Source: CAD feature listing. Evaluate the final solid. Frame: model axes, mm. Face numbers are marked on the shaded views. A direction names the side the tool comes from. Coordinates: 2 decimals unless noted, no trailing zeros. Order: outer loops, then holes, each group sorted by start corner. A loop starts at its lowest first (then second) coordinate and runs counter-clockwise, first axis right, second up.
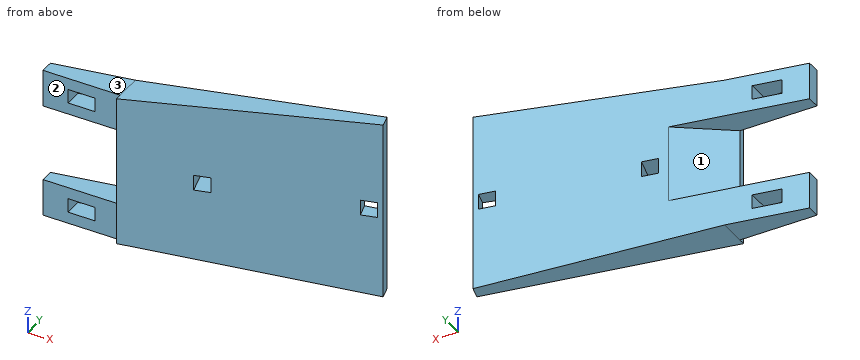
```python
from build123d import *

# Parameters (mm, degrees)
SALIENTE_EXTRUIR1_DEPTH     = 70
CORTAR_EXTRUIR1_START       = -26.44505645
CORTAR_EXTRUIR1_OUTLINE_W   = 30
CORTAR_EXTRUIR1_OUTLINE_H   = 30
CORTAR_EXTRUIR1_OUTLINE_W_2 = 10.5
CORTAR_EXTRUIR1_OUTLINE_H_2 = 5.5
CORTAR_EXTRUIR1_DEPTH       = 28.94505645
CROQUIS3_W                  = 6
CROQUIS3_H                  = 6
CORTAR_EXTRUIR2_DEPTH       = 118.634247959
CORTAR_EXTRUIR3_DEPTH       = 15
CORTAR_EXTRUIR3_DEPTH_BACK  = 15


# Read off the part's stored shape, not the designer's step: Cortar-Extruir1
with BuildPart() as part:
    # Croquis1 → Saliente-Extruir1 (new body)
    with BuildSketch(Plane.XY):
        Polygon((0, 0), (90, 24.115427319), (88.705904774, 28.94505645), (-30, 7.5), (-30, 2.5), (0, 2.5), align=None)
    extrude(amount=SALIENTE_EXTRUIR1_DEPTH)

    # Cortar-Extruir1 outline → Cortar-Extruir1 (cut)
    with BuildSketch(Plane.XZ.offset(-2.5).offset(CORTAR_EXTRUIR1_START)):
        Polygon((90, 0), (0, 5.5), (-30, 5.5), (-30, 0), align=None)
        with Locations((-15, 35)):
            Rectangle(CORTAR_EXTRUIR1_OUTLINE_W, CORTAR_EXTRUIR1_OUTLINE_H)
        Polygon((-30, 64.5), (0, 64.5), (90, 70), (-30, 70), align=None)
        with Locations((-15, 12.75)):
            Rectangle(CORTAR_EXTRUIR1_OUTLINE_W_2, CORTAR_EXTRUIR1_OUTLINE_H_2)
        with Locations((-15, 57.25)):
            Rectangle(CORTAR_EXTRUIR1_OUTLINE_W_2, CORTAR_EXTRUIR1_OUTLINE_H_2)
    extrude(amount=CORTAR_EXTRUIR1_DEPTH, mode=Mode.SUBTRACT)

    # Croquis3 → Cortar-Extruir2 (cut, through all)
    with BuildSketch(Plane(origin=(0, 0, 0), x_dir=(0.9659258262890692, 0.2588190451025179, 0), z_dir=(0.2588190451025179, -0.9659258262890692, 0))):
        with Locations((30, 35)):
            Rectangle(CROQUIS3_W, CROQUIS3_H)
        with Locations((88.174856237, 35)):
            Rectangle(CROQUIS3_W, CROQUIS3_H)
    extrude(amount=-CORTAR_EXTRUIR2_DEPTH, mode=Mode.SUBTRACT)

    # Croquis4 → Cortar-Extruir3 (cut, two sides: drawn at the far end of the back side and taken through both)
    with BuildSketch(Plane.XY.offset(35).offset(-CORTAR_EXTRUIR3_DEPTH_BACK)):
        Polygon((0, 2.5), (0, 12.919710963), (19.681407906, 16.475295703), align=None)
    extrude(amount=CORTAR_EXTRUIR3_DEPTH + CORTAR_EXTRUIR3_DEPTH_BACK, mode=Mode.SUBTRACT)


solid = part.part
```
1. Section query B-B on z = 52.5. Return loops of the section in (x, y), plus the area to 3 significant figures.
Findings:
outline: (-30, 2.5) - (0, 2.5) - (0, 0) - (90, 24.12) - (88.71, 28.95) - (-30, 7.5) - close
area: 1,040 mm2
2. Access query for the marked faces 1, 2 and 3. Directions: +Z, -Z, +X, -X, +Y, -Y. A direction counts if a zero-diameter tool reaches every point of the face in a straight line with its end or side. Return the directions, or none.
Findings:
face 1: -X, +Y
face 2: +Z, -Z, -X, -Y
face 3: +Z, -X, +Y, -Y
3. Pin query (flat end, axial travel): P1, Ø11, axis at x = -7, y = 10, coming from the +Z side; P2, Ø7, axis at x = -21.5, z = 10.5, coming from the -Y side; P3, Ø10, axis at x = -13.5, z = 57.5, coming from the +Y side. Return the tip coordinate at first contact, or that it passes through.
Findings:
P1: stops at z = 64.5
P2: stops at y = 2.5
P3: stops at y = 11.38
4. Section query A-A on x = -13. Return loops of the section in (y, z), plus the area to 3 significant figures.
Findings:
outline: (2.5, 5.5) - (10.57, 5.5) - (10.57, 10) - (2.5, 10) - close; (2.5, 15.5) - (10.57, 15.5) - (10.57, 20) - (2.5, 20) - close; (2.5, 50) - (10.57, 50) - (10.57, 54.5) - (2.5, 54.5) - close; (2.5, 60) - (10.57, 60) - (10.57, 64.5) - (2.5, 64.5) - close
area: 145 mm2
5. Ray query, line 1 (Z direction, x = -18, y = 5.5); line 2 (Y direction, x = 70.5, z = 53); line 3 (Y direction, x = 35, z = 41.5). Return the intervals inside material, ascending.
Findings:
line 1: z = 5.5 to 10, 15.5 to 20, 50 to 54.5, 60 to 64.5
line 2: y = 18.89 to 25.66
line 3: y = 9.38 to 19.24
6. Section query D-D on x = 24.5. Return loops of the section in (y, z).
Findings:
outline: (6.56, 4) - (17.35, 4) - (17.35, 32) - (12.88, 32) - (12.88, 38) - (17.35, 38) - (17.35, 66) - (6.56, 66) - close
7. Section query C-C on y = 15. Return loops of the section in (x, z).
Findings:
outline: (11.52, 4.8) - (55.98, 2.08) - (55.98, 67.92) - (11.52, 65.2) - (11.52, 50) - (17.6, 50) - (17.6, 20) - (11.52, 20) - close; hole (23.93, 32) - (30.14, 32) - (30.14, 38) - (23.93, 38) - close
